Answer from the drawing. Dimensions are ordinates in mm from the lowest x, y and z of the part. A direction names the side the tool comes from. Coordinates: 2 decimals unless noted, no trailing zeros. Order: outer loops, then holes, each group sorted by start corner. A loop starts at its lowest first (then second) coordinate and runs counter-clockwise, first axis right, second up. Notation, with made-up numbers: M -21.75,49.5 L -15.75,49.5 A22 ccw -15.75,83.5 Z; hole C 51.5,-23 d4. An arc over 180 degrees is marked long. Use a Markdown table: item, result.
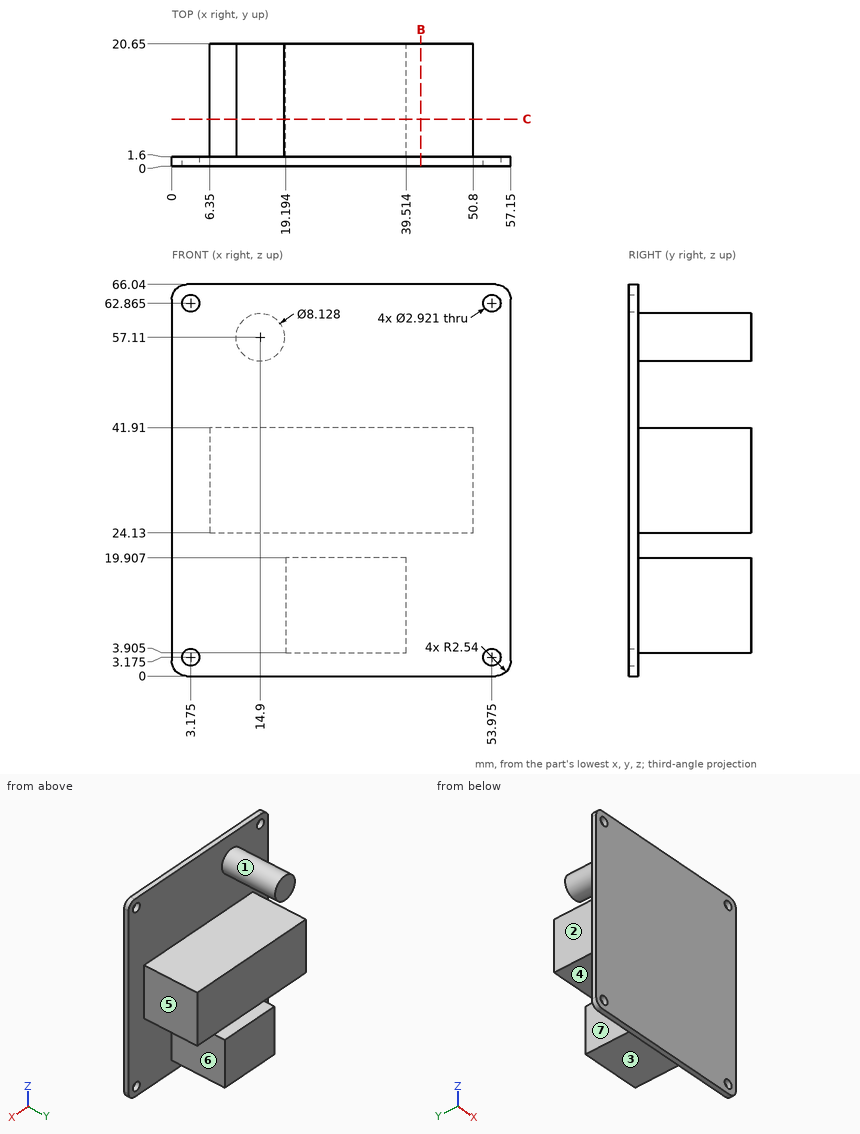
(1) A cutting plane is placed at B-B (x = 42). Determine the outline of the cut face in (y, z).
Conclusion:
| item | result |
|---|---|
| outline | M 0,0 L 1.6,0 L 1.6,24.13 L 20.65,24.13 L 20.65,41.91 L 1.6,41.91 L 1.6,66.04 L 0,66.04 Z |
(2) Which of the six approach directions +Z, -Z, +X, -X, +Y, -Y give full straight-line access (tool end or side, diameter ignored) to the marked faces 5, 6 and 7?
Conclusion:
| item | result |
|---|---|
| face 5 | +Z, -Z, +X, +Y |
| face 6 | -Z, +X, +Y |
| face 7 | -Z, -X, +Y |
(3) Determine the mould class of the marked faces 1, 2, 3 and 4 for opening direction Z: pulls with the +Z half, pulls with the -Z half, needs draft (parallel to the pull), parting line crosses it, or undercut.
Conclusion:
| item | result |
|---|---|
| face 1 | undercut |
| face 2 | needs draft |
| face 3 | pulls with the -Z half |
| face 4 | undercut |
(4) Straight lines are drawn through the part: L1, parallel to Z at x = 24, y = 8.25 (1 decimal); L2, parallel to Z at x = 53.5, y = 1 (1 decimal); L3, parallel to X at y = 9.25, z = 33.5. For each, find the intervals that lie inside material, in ascending order.
Conclusion:
| item | result |
|---|---|
| L1 | 3.9 to 19.9, 24.1 to 41.9 |
| L2 | 0 to 1.8, 4.6 to 61.5, 64.2 to 66 |
| L3 | 6.35 to 50.8 |
(5) Given P1, Ø5.5, axis at x = 34.5, y = 9, coming from the +Z side; P2, Ø2.5, axis at x = 3.175, z = 62.865, coming from the -Y side; P3, Ø5, axis at y = 12.5, z = 12.5, coming from the -X side; P4, Ø8, axis at x = 49.5, y = 5, coming from the +Z side, each flat-ended and moving along its own axis, determine where each tip first touches the part or whether it passes through.
Conclusion:
| item | result |
|---|---|
| P1 | z = 41.91 |
| P2 | through |
| P3 | x = 19.19 |
| P4 | z = 66.04 |
(6) A cutting plane is placed at C-C (y = 8). Give the number of separate pieces and of enclosed holes in the cut face, then the cut area to 3 significant figures.
Conclusion:
| item | result |
|---|---|
| separate pieces | 3 |
| enclosed holes | 0 |
| area | 1,170 mm2 |
